Here's how the part is built. I have some questions about the finished solid (model axes, mm). A direction names the side the tool comes from. Round coordinates to 2 decimals unless told otherwise and drop trailing zeros. Loops run counter-clockwise (first coordinate to the right, second up) from the corner with the lowest first, then second, coordinate; pieces in that order, holes last. Notation, with made-up numbers: M -2.5,-0.5 L 53.5,-0.5 A13 ccw 53.5,11.5 Z; hole C 34,32 d6. An arc over 180 degrees is marked long. Use a Markdown table: item, result.
from build123d import *

# Parameters (mm, degrees)
F0_W         = 2.3
F0_H         = 3.2
F1_DEPTH     = 1.8
F0_W_2       = 8.7
F0_H_2       = 2.5
F2_DEPTH     = 0.9
F0_W_3       = 0.6
F3_DEPTH     = 1
F4_DEPTH     = 0.8
F5_DEPTH     = 0.8
F6_T4_DEPTH  = 9.5863757687
F6_T10_DEPTH = 9.5863757687
F6_T16_DEPTH = 17.1863757687
F6_T23_DEPTH = 17.1863757687
F6_T31_DEPTH = 9.5863757687
F6_T37_DEPTH = 9.5863757687
F7_T1_DEPTH  = 6.6641016151
F7_T3_DEPTH  = 6.7
F8_T1_DEPTH  = 8.5
F8_T3_DEPTH  = 20.7
F8_T5_DEPTH  = 8.5
F8_T7_DEPTH  = 20.6749371855
F0_W_4       = 1.5
F0_H_3       = 1.3
F9_DEPTH     = 0.2
F10_DEPTH    = 1.1
F11_R        = 0.64999
F12_R        = 0.64999


# Not quite as in the source:
# - a fillet or chamfer that OpenCascade refuses, or shapes differently, is made with other operations: its cross-section is extruded or revolved along the edge and cut away or added
# - a fillet or chamfer is up to 0.001 mm smaller than in the source, because OpenCascade refuses the exact size


with BuildPart() as f1:
    # F0 (on Top) → F1 (new body)
    with BuildSketch(Plane.XY):
        Polygon((8.8998297817, -13.0360927206), (-6.8001702183, -13.0360927206), (-6.8001702183, -16.0360927206), (-6.8001702183, -17.0360927206), (-6.8001702183, -18.3360927206), (-6.8001702183, -19.0360927206), (-3.3001702183, -19.0360927206), (-3.3001702183, -16.5360927206), (5.3998297817, -16.5360927206), (5.3998297817, -19.0360927206), (8.8998297817, -19.0360927206), (8.8998297817, -18.3360927206), (8.8998297817, -17.0360927206), align=None)
        Polygon((-4.2001702183, 41.7639072794), (-6.8001702183, 41.7639072794), (-6.8001702183, 38.2639072794), (-4.5001702183, 38.2639072794), (-4.5001702183, 35.0639072794), (-6.8001702183, 35.0639072794), (-6.8001702183, -13.0360927206), (8.8998297817, -13.0360927206), (8.8998297817, 35.0639072794), (6.5998297817, 35.0639072794), (6.5998297817, 38.2639072794), (8.8998297817, 38.2639072794), (8.8998297817, 41.7639072794), (6.2998297817, 41.7639072794), (6.2998297817, 38.8639072794), (-4.2001702183, 38.8639072794), align=None)
        with Locations((7.7498297817, 36.6639072794)):
            Rectangle(F0_W, F0_H)
        with Locations((-5.6501702183, 36.6639072794)):
            Rectangle(F0_W, F0_H)
    extrude(amount=F1_DEPTH)

    # F0 (on Top) → F2 (join)
    with BuildSketch(Plane.XY):
        with Locations((1.0498297817, -17.7860927206)):
            Rectangle(F0_W_2, F0_H_2)
        Polygon((8.8998297817, -13.0360927206), (-6.8001702183, -13.0360927206), (-6.8001702183, -16.0360927206), (-6.8001702183, -17.0360927206), (-6.8001702183, -18.3360927206), (-6.8001702183, -19.0360927206), (-3.3001702183, -19.0360927206), (-3.3001702183, -16.5360927206), (5.3998297817, -16.5360927206), (5.3998297817, -19.0360927206), (8.8998297817, -19.0360927206), (8.8998297817, -18.3360927206), (8.8998297817, -17.0360927206), align=None)
    extrude(amount=-F2_DEPTH)

    # F0 (on Top) → F3 (join)
    with BuildSketch(Plane.XY):
        with Locations((7.7498297817, 36.6639072794)):
            Rectangle(F0_W, F0_H)
        with Locations((9.1998297817, 36.6639072794)):
            Rectangle(F0_W_3, F0_H)
        with Locations((-5.6501702183, 36.6639072794)):
            Rectangle(F0_W, F0_H)
        with Locations((-7.1001702183, 36.6639072794)):
            Rectangle(F0_W_3, F0_H)
    extrude(amount=-F3_DEPTH)

    # F0 (on Top) → F4 (join)
    with BuildSketch(Plane.XY):
        with Locations((9.1998297817, 36.6639072794)):
            Rectangle(F0_W_3, F0_H)
        with Locations((-7.1001702183, 36.6639072794)):
            Rectangle(F0_W_3, F0_H)
    extrude(amount=F4_DEPTH)

    # F0 (on Top) → F5 (join)
    with BuildSketch(Plane.XY):
        with Locations((1.0498297817, -17.7860927206)):
            Rectangle(F0_W_2, F0_H_2)
    extrude(amount=F5_DEPTH)

    # F6: chamfer of 1.3 on 3 edges, made by hand


with BuildPart() as f6_tool2:
    # F6_s3 → F6_t4 (new body)
    with BuildSketch(Plane.XZ.offset(-45.1070951637)):
        Polygon((7.5998297817, 0), (6.2998297817, 1.3), (6.2998297817, 0), align=None)
    extrude(amount=F6_T4_DEPTH)

    split(bisect_by=Plane.XZ.offset(-38.2639072794), keep=Keep.BOTTOM)

    split(bisect_by=Plane(origin=(0, 18.7819536397, -18.7819536397), x_dir=(1, 0, 0), z_dir=(0, 0.7071067812, -0.7071067812)), keep=Keep.TOP)


with BuildPart() as f1_1:
    add(f1.part)

    # F6_t1: cut F6_tool2
    add(f6_tool2.part, mode=Mode.SUBTRACT)


with BuildPart() as f6_tool8:
    # F6_s9 → F6_t10 (new body)
    with BuildSketch(Plane.XZ.offset(-45.1070951637)):
        Polygon((7.5998297817, 0), (6.2998297817, 1.3), (6.2998297817, 0), align=None)
    extrude(amount=F6_T10_DEPTH)

    split(bisect_by=Plane.YZ.offset(6.5998297817), keep=Keep.BOTTOM)

    split(bisect_by=Plane(origin=(0, 18.7819536397, -18.7819536397), x_dir=(1, 0, 0), z_dir=(0, 0.7071067812, -0.7071067812)), keep=Keep.TOP)


with BuildPart() as f1_2:
    add(f1_1.part)

    # F6_t7: cut F6_tool8
    add(f6_tool8.part, mode=Mode.SUBTRACT)


with BuildPart() as f6_tool14:
    # F6_s15 → F6_t16 (new body)
    with BuildSketch(Plane.YZ.offset(9.6430176661)):
        Polygon((37.5639072794, 0), (38.8639072794, 1.3), (38.8639072794, 0), align=None)
    extrude(amount=-F6_T16_DEPTH)

    split(bisect_by=Plane.XZ.offset(-38.2639072794), keep=Keep.BOTTOM)

    split(bisect_by=Plane(origin=(-2.7500851092, 0, 2.7500851092), x_dir=(0, 1, 0), z_dir=(0.7071067812, 0, -0.7071067812)), keep=Keep.TOP)

    split(bisect_by=Plane(origin=(3.7999148908, 0, 3.7999148908), x_dir=(0, 1, 0), z_dir=(-0.7071067812, 0, -0.7071067812)), keep=Keep.TOP)


with BuildPart() as f1_3:
    add(f1_2.part)

    # F6_t13: cut F6_tool14
    add(f6_tool14.part, mode=Mode.SUBTRACT)


with BuildPart() as f6_tool21:
    # F6_s22 → F6_t23 (new body)
    with BuildSketch(Plane.YZ.offset(9.6430176661)):
        Polygon((37.5639072794, 0), (38.8639072794, 1.3), (38.8639072794, 0), align=None)
    extrude(amount=-F6_T23_DEPTH)

    split(bisect_by=Plane.YZ.offset(6.5998297817), keep=Keep.BOTTOM)

    split(bisect_by=Plane.YZ.offset(-4.5001702183), keep=Keep.TOP)

    split(bisect_by=Plane(origin=(-2.7500851092, 0, 2.7500851092), x_dir=(0, 1, 0), z_dir=(0.7071067812, 0, -0.7071067812)), keep=Keep.TOP)

    split(bisect_by=Plane(origin=(3.7999148908, 0, 3.7999148908), x_dir=(0, 1, 0), z_dir=(-0.7071067812, 0, -0.7071067812)), keep=Keep.TOP)


with BuildPart() as f1_4:
    add(f1_3.part)

    # F6_t20: cut F6_tool21
    add(f6_tool21.part, mode=Mode.SUBTRACT)


with BuildPart() as f6_tool29:
    # F6_s30 → F6_t31 (new body)
    with BuildSketch(Plane.XZ.offset(-35.520719395)):
        Polygon((-5.5001702183, 0), (-4.2001702183, 1.3), (-4.2001702183, 0), align=None)
    extrude(amount=-F6_T31_DEPTH)

    split(bisect_by=Plane.YZ.offset(-4.5001702183), keep=Keep.TOP)

    split(bisect_by=Plane(origin=(0, 18.7819536397, -18.7819536397), x_dir=(1, 0, 0), z_dir=(0, 0.7071067812, -0.7071067812)), keep=Keep.TOP)


with BuildPart() as f1_5:
    add(f1_4.part)

    # F6_t28: cut F6_tool29
    add(f6_tool29.part, mode=Mode.SUBTRACT)


with BuildPart() as f6_tool35:
    # F6_s36 → F6_t37 (new body)
    with BuildSketch(Plane.XZ.offset(-35.520719395)):
        Polygon((-5.5001702183, 0), (-4.2001702183, 1.3), (-4.2001702183, 0), align=None)
    extrude(amount=-F6_T37_DEPTH)

    split(bisect_by=Plane.XZ.offset(-38.2639072794), keep=Keep.BOTTOM)

    split(bisect_by=Plane(origin=(0, 18.7819536397, -18.7819536397), x_dir=(1, 0, 0), z_dir=(0, 0.7071067812, -0.7071067812)), keep=Keep.TOP)


with BuildPart() as f1_6:
    add(f1_5.part)

    # F6_t34: cut F6_tool35
    add(f6_tool35.part, mode=Mode.SUBTRACT)

    # F7: fillet of radius 0.7 on 6 edges, made by hand

    # F7_s2 → F7_t1 (cut)
    with BuildSketch(Plane.XZ.offset(-39.9959580869)):
        with BuildLine():
            ThreePointArc((-7.4001702183, 0.107179677), (-7.2293204805, 0.5654372465), (-6.8001702183, 0.8))
            Line((-6.8001702183, 0.8), (-7.4001702183, 0.8))
            Line((-7.4001702183, 0.8), (-7.4001702183, 0.107179677))
        make_face()
        with BuildLine():
            ThreePointArc((9.4998297817, 0.107179677), (9.3289800439, 0.5654372465), (8.8998297817, 0.8))
            Line((8.8998297817, 0.8), (9.4998297817, 0.8))
            Line((9.4998297817, 0.8), (9.4998297817, 0.107179677))
        make_face()
    extrude(amount=F7_T1_DEPTH, mode=Mode.SUBTRACT)

    # F7_s4 → F7_t3 (cut)
    with BuildSketch(Plane.XZ.offset(-40.0139072794)):
        with BuildLine():
            ThreePointArc((-6.7001702183, -1), (-7.1951449651, -0.7949747468), (-7.4001702183, -0.3))
            Line((-7.4001702183, -0.3), (-7.4001702183, -1))
            Line((-7.4001702183, -1), (-6.7001702183, -1))
        make_face()
        with BuildLine():
            ThreePointArc((-5.2001702183, -1), (-4.7051954715, -0.7949747468), (-4.5001702183, -0.3))
            Line((-4.5001702183, -0.3), (-4.5001702183, -1))
            Line((-4.5001702183, -1), (-5.2001702183, -1))
        make_face()
        with BuildLine():
            ThreePointArc((6.5998297817, -0.3), (6.8048550349, -0.7949747468), (7.2998297817, -1))
            Line((7.2998297817, -1), (6.5998297817, -1))
            Line((6.5998297817, -1), (6.5998297817, -0.3))
        make_face()
        with BuildLine():
            ThreePointArc((8.7998297817, -1), (9.2948045285, -0.7949747468), (9.4998297817, -0.3))
            Line((9.4998297817, -0.3), (9.4998297817, -1))
            Line((9.4998297817, -1), (8.7998297817, -1))
        make_face()
    extrude(amount=F7_T3_DEPTH, mode=Mode.SUBTRACT)

    # F8: fillet of radius 1 on 4 edges, made by hand

    # F8_s2 → F8_t1 (cut)
    with BuildSketch(Plane.YZ.offset(-9.3001702183)):
        with BuildLine():
            ThreePointArc((-19.0360927206, 0.8), (-18.7431995018, 1.5071067812), (-18.0360927206, 1.8))
            Line((-18.0360927206, 1.8), (-19.0360927206, 1.8))
            Line((-19.0360927206, 1.8), (-19.0360927206, 0.8))
        make_face()
    extrude(amount=F8_T1_DEPTH, mode=Mode.SUBTRACT)

    # F8_s4 → F8_t3 (cut)
    with BuildSketch(Plane.YZ.offset(-9.3001702183)):
        with BuildLine():
            ThreePointArc((-19.0360927206, 0.1), (-18.7431995018, -0.6071067812), (-18.0360927206, -0.9))
            Line((-18.0360927206, -0.9), (-19.0360927206, -0.9))
            Line((-19.0360927206, -0.9), (-19.0360927206, 0.1))
        make_face()
    extrude(amount=F8_T3_DEPTH, mode=Mode.SUBTRACT)

    # F8_s6 → F8_t5 (cut)
    with BuildSketch(Plane.YZ.offset(2.8998297817)):
        with BuildLine():
            ThreePointArc((-19.0360927206, 0.8), (-18.7431995018, 1.5071067812), (-18.0360927206, 1.8))
            Line((-18.0360927206, 1.8), (-19.0360927206, 1.8))
            Line((-19.0360927206, 1.8), (-19.0360927206, 0.8))
        make_face()
    extrude(amount=F8_T5_DEPTH, mode=Mode.SUBTRACT)

    # F8_s8 → F8_t7 (cut)
    with BuildSketch(Plane.YZ.offset(-9.2876388111)):
        with BuildLine():
            ThreePointArc((-14.0310801578, -0.9), (-13.3602597645, -0.6416198487), (-13.0360927206, 0))
            Line((-13.0360927206, 0), (-13.0360927206, -0.9))
            Line((-13.0360927206, -0.9), (-14.0310801578, -0.9))
        make_face()
    extrude(amount=F8_T7_DEPTH, mode=Mode.SUBTRACT)

    # F0 (on Top) → F9 (join)
    with BuildSketch(Plane.XY):
        with Locations((-7.5501702183, -17.6860927206)):
            Rectangle(F0_W_4, F0_H_3)
        with Locations((9.6498297817, -17.6860927206)):
            Rectangle(F0_W_4, F0_H_3)
    extrude(amount=-F9_DEPTH)

    # F0 (on Top) → F10 (join)
    with BuildSketch(Plane.XY):
        with Locations((-7.5501702183, -17.6860927206)):
            Rectangle(F0_W_4, F0_H_3)
        with Locations((9.6498297817, -17.6860927206)):
            Rectangle(F0_W_4, F0_H_3)
    extrude(amount=F10_DEPTH)

    # F11 (radius 0.65 in the source; OpenCascade refuses exactly that, so slightly less here)
    f11_edges = [f1_6.edges().sort_by_distance(p)[0] for p in [
        (9.64983, -17.036093, 1.1),
        (9.64983, -18.336093, 1.1),
    ]]
    fillet(f11_edges, radius=F11_R)

    # F12 (radius 0.65 in the source; OpenCascade refuses exactly that, so slightly less here)
    f12_edges = [f1_6.edges().sort_by_distance(p)[0] for p in [
        (9.64983, -18.336093, -0.2),
        (9.64983, -17.036093, -0.2),
        (-7.55017, -18.336093, -0.2),
        (-7.55017, -17.036093, -0.2),
        (-7.55017, -18.336093, 1.1),
        (-7.55017, -17.036093, 1.1),
    ]]
    fillet(f12_edges, radius=F12_R)


solid = f1_6.part
1. I need wall thicknesses on probe 1 along X at (y, z) = (38.5, 1.1); probe 2 along Y at (x, z) = (1.25, 1.35); probe 3 along Z at (x, y) = (-6.5, 28.5). Which ranges of each line are inside material? Lowest first, please. Write a range as from..to.
Answer sheet:
| item | result |
|---|---|
| probe 1 | -6.8..8.9 |
| probe 2 | -16.54..38.86 |
| probe 3 | 0..1.8 |
2. Which directions (+Z, -Z, +X, -X, +Y, -Y) give clear straight access to the entire face, cutting with the end or side of a thin tool? Please do faces 5 (the face through (7, 40, 0.6)), 6 (the face through (-6, 35.064, -0.3)), 7 (the face through (0.94, -13.37, -0.65)).
Answer sheet:
| item | result |
|---|---|
| face 5 | -Z, +Y |
| face 6 | -Z, -X |
| face 7 | -Z, +X, -X |
3. Imagine slicing it at B-B, the plane y = -8. Write out the boundary of the cut face in (x, z).
Answer sheet:
| item | result |
|---|---|
| outline | M -6.8,0 L 8.9,0 L 8.9,1.8 L -6.8,1.8 Z |
4. For pin 1 Ø0.5 at (y, z) = (-17, 1.5) entering from -X, with a flat end and sliding along its axis, tell me the tip position at first contact or that it passes through.
Answer sheet:
| item | result |
|---|---|
| pin 1 | x = -6.8 |
5. Imagine slicing it at A-A, the plane x = 3.25. Write out the boundary of the cut face in (y, z), then the cut area to 3 significant figures.
Answer sheet:
| item | result |
|---|---|
| outline | M -19.04,0.1 A1 ccw -18.04,-0.9 L -14.03,-0.9 A1 ccw -13.04,0 L 37.56,0 L 38.86,1.3 L 38.86,1.8 L -16.54,1.8 L -16.54,0.8 L -19.04,0.8 Z |
| area | 106 mm2 |
6. We'd pull the mould along X, two halves only. Please class faces 1 (the face through (-6, 41.764, 1)), 2 (the face through (10.4, -17.7, 0.5)), 3 (the face through (-5.9, 38.264, -0.3)), 4 (the face through (-6.8, 12, 1)): +X half, -X half, draft (parallel to the pull), parting line (faces both ways), or undercut.
Answer sheet:
| item | result |
|---|---|
| face 1 | draft |
| face 2 | +X half |
| face 3 | undercut |
| face 4 | -X half |
